```python
from build123d import *

# Parameters (mm, degrees)
SKETCH1_R           = 45
SKETCH1_R_2         = 30
SKETCH1_R_3         = 1.75
BOSS_EXTRUDE1_DEPTH = 6
SKETCH2_R           = 36
CUT_EXTRUDE1_DEPTH  = 3
SKETCH3_R           = 3.25
CUT_EXTRUDE2_DEPTH  = 3


with BuildPart() as part:
    # Sketch1 → Boss-Extrude1 (new body)
    with BuildSketch(Plane(origin=(0, 0, 0), x_dir=(1, 0, 0), z_dir=(0, 1, 0))):
        with Locations(Location((0, 0, 0), (0, 0, 270))):
            Circle(SKETCH1_R)
        with Locations(Location((0, 0, 0), (0, 0, 270))):
            Circle(SKETCH1_R_2, mode=Mode.SUBTRACT)
        with Locations(Location((0, 40, 0), (0, 0, 270))):
            Circle(SKETCH1_R_3, mode=Mode.SUBTRACT)
        with Locations(Location((20, 34.641016151, 0), (0, 0, 270))):
            Circle(SKETCH1_R_3, mode=Mode.SUBTRACT)
        with Locations(Location((34.641016151, 20, 0), (0, 0, 270))):
            Circle(SKETCH1_R_3, mode=Mode.SUBTRACT)
        with Locations(Location((40, 0, 0), (0, 0, 270))):
            Circle(SKETCH1_R_3, mode=Mode.SUBTRACT)
        with Locations(Location((34.641016151, -20, 0), (0, 0, 270))):
            Circle(SKETCH1_R_3, mode=Mode.SUBTRACT)
        with Locations(Location((20, -34.641016151, 0), (0, 0, 270))):
            Circle(SKETCH1_R_3, mode=Mode.SUBTRACT)
        with Locations(Location((0, -40, 0), (0, 0, 270))):
            Circle(SKETCH1_R_3, mode=Mode.SUBTRACT)
        with Locations(Location((-20, -34.641016151, 0), (0, 0, 270))):
            Circle(SKETCH1_R_3, mode=Mode.SUBTRACT)
        with Locations(Location((-34.641016151, -20, 0), (0, 0, 270))):
            Circle(SKETCH1_R_3, mode=Mode.SUBTRACT)
        with Locations(Location((-40, 0, 0), (0, 0, 270))):
            Circle(SKETCH1_R_3, mode=Mode.SUBTRACT)
        with Locations(Location((-34.641016151, 20, 0), (0, 0, 270))):
            Circle(SKETCH1_R_3, mode=Mode.SUBTRACT)
        with Locations(Location((-20, 34.641016151, 0), (0, 0, 270))):
            Circle(SKETCH1_R_3, mode=Mode.SUBTRACT)
    extrude(amount=BOSS_EXTRUDE1_DEPTH)

    # Sketch2 → Cut-Extrude1 (cut)
    with BuildSketch(Plane.XZ):
        with Locations(Location((0, 0, 0), (0, 0, 270))):
            Circle(SKETCH2_R)
    extrude(amount=-CUT_EXTRUDE1_DEPTH, mode=Mode.SUBTRACT)

    # Sketch3 → Cut-Extrude2 (cut)
    with BuildSketch(Plane(origin=(0, 6, 0), x_dir=(1, 0, 0), z_dir=(0, 1, 0))):
        with Locations(Location((40, 0, 0), (0, 0, 270))):
            Circle(SKETCH3_R)
        with Locations(Location((34.641016151, -20, 0), (0, 0, 270))):
            Circle(SKETCH3_R)
        with Locations(Location((20, -34.641016151, 0), (0, 0, 270))):
            Circle(SKETCH3_R)
        with Locations(Location((0, -40, 0), (0, 0, 270))):
            Circle(SKETCH3_R)
        with Locations(Location((-20, -34.641016151, 0), (0, 0, 270))):
            Circle(SKETCH3_R)
        with Locations(Location((-34.641016151, -20, 0), (0, 0, 270))):
            Circle(SKETCH3_R)
        with Locations(Location((-40, 0, 0), (0, 0, 270))):
            Circle(SKETCH3_R)
        with Locations(Location((-34.641016151, 20, 0), (0, 0, 270))):
            Circle(SKETCH3_R)
        with Locations(Location((-20, 34.641016151, 0), (0, 0, 270))):
            Circle(SKETCH3_R)
        with Locations(Location((0, 40, 0), (0, 0, 270))):
            Circle(SKETCH3_R)
        with Locations(Location((20, 34.641016151, 0), (0, 0, 270))):
            Circle(SKETCH3_R)
        with Locations(Location((34.641016151, 20, 0), (0, 0, 270))):
            Circle(SKETCH3_R)
    extrude(amount=-CUT_EXTRUDE2_DEPTH, mode=Mode.SUBTRACT)


solid = part.part
```
Check sheet for the modelled part. Datum: model origin and axes. Units: mm. A direction names the side the tool comes from. Give positions to 0.01 mm unless a question says otherwise; leave off trailing zeros. Write each loop counter-clockwise with the first axis right and the second up, starting at its lowest first coordinate (ties: lowest second). Pieces come first, ordered by that corner, then holes. Notation, with made-up numbers: (32, 44.25) -> (70, 44.25) arc R19 cw to (70, 68.25) -> close; hole circle Ø6 at (71.5, 47). An arc over 180 degrees is marked (long way). Use CSV: the item, a comma, the result in double quotes. Start each with the question number.
Q1. Cross-section at C-C on z = 40. Enter the section's corners in (x, y).
Q2. Scan lines: line 1 along X through (y, z) = (4.35, 36); line 2 along X through (y, z) = (1.8, -20); line 3 along Z through (x, y) = (22, 5.25). Record each from-to range of solid material in increasing order.
Q3. Cross-section at A-A on z = 0. Enter the section's corners in (x, y), and give its area (3 significant figures).
Q4. Cross-section at D-D on x = -20. Enter the section's corners in (y, z), and give its area (3 significant figures).
Q5. Tool access check on faces 1 (the cylindrical face through (36.827, 4.521, -0.705)), 2 (the cylindrical face through (-33.46, 1.48, -21.29)). Record the directions out of +Z, -Z, +X, -X, +Y, -Y that give a thin tool (end or side, any length) a straight path to the whole face; none if there is none.
Q6. Release check for a two-part mould opening along Z. For faces 3 (the cylindrical face through (-18.82, 1.48, 33.35)), 4 (the cylindrical face through (-17.235, 2.958, 41.569)) record: +Z half, -Z half, draft (parallel to the pull), parting line (faces both ways), or undercut.
Q7. Depth check by flat-ended pin: P1, Ø4, axis at x = -20, z = 34.64, coming from the +Y side. Enter the tip coordinate at first touch or a pass-through.
Q8. Cross-section at B-B on x = 40. Enter the section's corners in (y, z), and give its area (3 significant figures).
Working result:
1,outline,"(-20.62, 0) -> (-1.75, 0) -> (-1.75, 3) -> (-3.25, 3) -> (-3.25, 6) -> (-20.62, 6) -> close; (1.75, 0) -> (20.62, 0) -> (20.62, 6) -> (3.25, 6) -> (3.25, 3) -> (1.75, 3) -> close"
2,line 1,"x = -27 to -22.95, -17.05 to 17.05, 22.95 to 27"
2,line 2,"x = -40.31 to -36.39, -32.89 to -29.93, 29.93 to 32.89, 36.39 to 40.31"
2,line 3,"z = -39.26 to -37.2, -32.08 to -20.4, 20.4 to 32.08, 37.2 to 39.26"
3,outline,"(-45, 0) -> (-41.75, 0) -> (-41.75, 3) -> (-43.25, 3) -> (-43.25, 6) -> (-45, 6) -> close; (-38.25, 0) -> (-36, 0) -> (-36, 3) -> (-30, 3) -> (-30, 6) -> (-36.75, 6) -> (-36.75, 3) -> (-38.25, 3) -> close; (30, 3) -> (36, 3) -> (36, 0) -> (38.25, 0) -> (38.25, 3) -> (36.75, 3) -> (36.75, 6) -> (30, 6) -> close; (41.75, 0) -> (45, 0) -> (45, 6) -> (43.25, 6) -> (43.25, 3) -> (41.75, 3) -> close"
3,area,"84.0 mm^2"
4,outline,"(0, -40.31) -> (6, -40.31) -> (6, -37.89) -> (3, -37.89) -> (3, -36.39) -> (0, -36.39) -> close; (0, -32.89) -> (3, -32.89) -> (3, -31.39) -> (6, -31.39) -> (6, -22.36) -> (3, -22.36) -> (3, -29.93) -> (0, -29.93) -> close; (0, 29.93) -> (3, 29.93) -> (3, 22.36) -> (6, 22.36) -> (6, 31.39) -> (3, 31.39) -> (3, 32.89) -> (0, 32.89) -> close; (0, 36.39) -> (3, 36.39) -> (3, 37.89) -> (6, 37.89) -> (6, 40.31) -> (0, 40.31) -> close"
4,area,"110 mm^2"
5,face 1,"+Y"
5,face 2,"+Y, -Y"
6,face 3,"undercut"
6,face 4,"parting line"
7,P1,"stops at y = 3"
8,outline,"(0, -20.62) -> (6, -20.62) -> (6, -3.25) -> (3, -3.25) -> (3, -1.75) -> (0, -1.75) -> close; (0, 1.75) -> (3, 1.75) -> (3, 3.25) -> (6, 3.25) -> (6, 20.62) -> (0, 20.62) -> close"
8,area,"217 mm^2"
